Here's the drawing with two shaded views (mm, measured from the low corner). I have some questions. Round coordinates to 2 decimals unless told otherwise and drop trailing zeros. Loops run counter-clockwise (first coordinate to the right, second up) from the corner with the lowest first, then second, coordinate; pieces in that order, holes last.
(1) If I drill on line 1 along Z through (x, y) = (60, 0.55); line 2 along X through (y, z) = (0.5, 29.5); line 3 along X through (y, z) = (0.25, 31.5), over which ranges is the centre line in solid material (lowest first)?
(2) I want a section at C-C on y = 0.7. Write out the boundary of the cut face in (x, z), plus the area to 3 significant figures.
(3) I want a section at D-D on z = 28. Write out the boundary of the cut face in (x, y), plus the area to 3 significant figures.
(4) I want a section at B-B on z = 32. Write out the boundary of the cut face in (x, y), plus the area to 3 significant figures.
(5) I want a section at A-A on x = 78.5. Write out the boundary of the cut face in (y, z), plus the area to 3 significant figures.
(6) Will this pin go through, and if not, where does the flat tip stop? pin 1 Ø0.6 at (x, y) = (19.5, 1) entering from +Z.
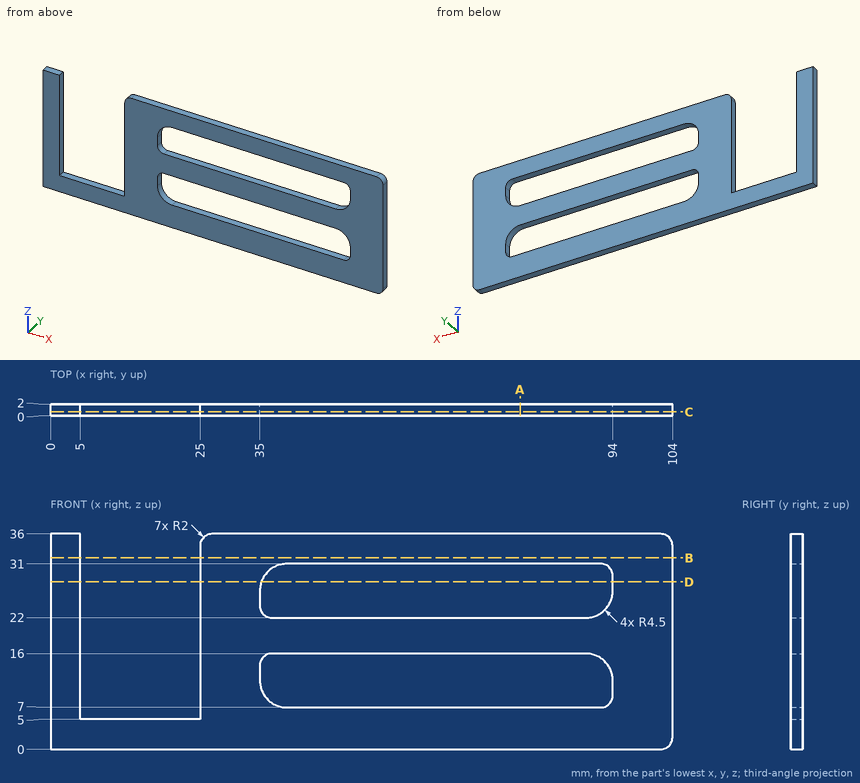
Filled sheet:
1. line 1: z = 0 to 7, 16 to 22, 31 to 36
1. line 2: x = 0 to 5, 25 to 36.15, 93.94 to 104
1. line 3: x = 0 to 5, 25 to 104
2. outline: (0, 0) - (102, 0) arc R2 ccw to (104, 2) - (104, 34) arc R2 ccw to (102, 36) - (27, 36) arc R2 ccw to (25, 34) - (25, 5) - (5, 5) - (5, 36) - (0, 36) - close; hole (35, 11.5) arc R4.5 ccw to (39.5, 7) - (92, 7) arc R2 ccw to (94, 9) - (94, 11.5) arc R4.5 ccw to (89.5, 16) - (37, 16) arc R2 ccw to (35, 14) - close; hole (35, 24) arc R2 ccw to (37, 22) - (89.5, 22) arc R4.5 ccw to (94, 26.5) - (94, 29) arc R2 ccw to (92, 31) - (39.5, 31) arc R4.5 ccw to (35, 26.5) - close
2. area: 2,080 mm2
3. outline: (0, 0) - (5, 0) - (5, 2) - (0, 2) - close; (25, 0) - (35.26, 0) - (35.26, 2) - (25, 2) - close; (94, 0) - (104, 0) - (104, 2) - (94, 2) - close
3. area: 50.5 mm2
4. outline: (0, 0) - (5, 0) - (5, 2) - (0, 2) - close; (25, 0) - (104, 0) - (104, 2) - (25, 2) - close
4. area: 168 mm2
5. outline: (0, 0) - (2, 0) - (2, 7) - (0, 7) - close; (0, 16) - (2, 16) - (2, 22) - (0, 22) - close; (0, 31) - (2, 31) - (2, 36) - (0, 36) - close
5. area: 36.0 mm2
6. pin 1: stops at z = 5
